Can you work these out from the model? Positions are in its coordinate system, mm. Face numbers are marked on the shaded views. Give positions to 0.01 mm unless a question says otherwise; leave off trailing zeros. Order: outer loops, then holes, each group sorted by start corner. A loop starts at its lowest first (then second) coordinate and runs counter-clockwise, first axis right, second up. Notation, with made-up numbers: (-5.5, -28.5) - (20.5, -28.5) arc R22 ccw to (20.5, -19.5) - close; hole circle Ø7 at (42, -25). An arc over 180 degrees is marked (long way). Use one line per item in the form item = value. Start each with the question number.
1) Suppose I cut it at A-A, the plane x = 0. Write out the boundary of the cut face in (y, z).
2) Suppose I cut it at B-B, the plane y = 43. Write out the boundary of the cut face in (x, z), and give its area (3 significant figures).
3) For pin 1 (2 mm diameter, centred on x = 5, y = 123, fed in from -Z); pin 2 (5 mm diameter, centred on y = 103.5, z = -5.5, fed in from -X), each with a flat end and sliding along its axis, tell me the tip position at first contact or that it passes through.
4) We'd pull the mould along Z, two halves only. Please class the marked faces 1 and 2: released by +Z, released by -Z, zero draft, split by the parting line, or undercut.
5) Suppose I cut it at C-C, the plane z = -2.5. Write out the boundary of the cut face in (x, y).
6) Please list where these lines run through material, in increasing order: probe 1 along X at (y, z) = (132, -0.25); probe 2 along Z at (x, y) = (-0.25, 47); probe 3 along X at (y, z) = (40, -1.5).
```python
from build123d import *

# Parameters (mm, degrees)
SEMICIRCULAR_TUBE_DEPTH = 170
FILLET_EDGES_R          = 1.1


with BuildPart() as part:
    # Sketch1 → semicircular tube (new body)
    with BuildSketch(Plane(origin=(0, 0, 0), x_dir=(1, 0, 0), z_dir=(0, 1, 0))):
        with BuildLine():
            Line((-9.35, 0), (-9.35, -3.5))
            Line((-9.35, -3.5), (9.35, -3.5))
            Line((9.35, -3.5), (9.35, 0))
            ThreePointArc((9.35, 0), (0, 9.35), (-9.35, 0))
        make_face()
        with BuildLine():
            Line((-6.35, 0), (6.35, 0))
            ThreePointArc((6.35, 0), (0, 6.35), (-6.35, 0))
        make_face(mode=Mode.SUBTRACT)
    extrude(amount=SEMICIRCULAR_TUBE_DEPTH)

    # fillet edges
    fillet_edges_edges = [part.edges().sort_by_distance(p)[0] for p in [
        (9.35, 85, 3.5),
        (-9.35, 85, 3.5),
    ]]
    fillet(fillet_edges_edges, radius=FILLET_EDGES_R)


solid = part.part
```
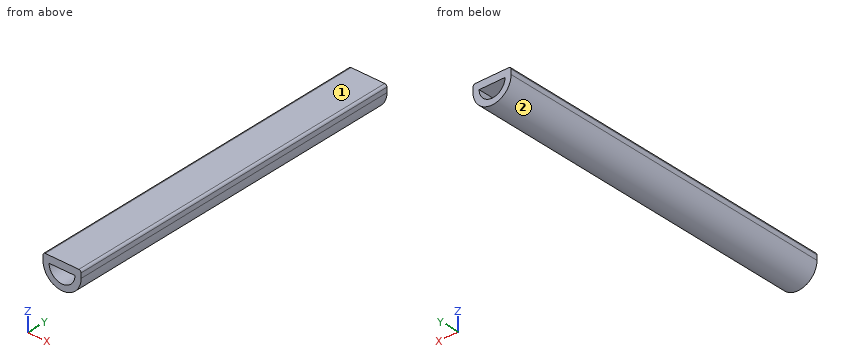
Result sheet:
q1.outline = (0, -9.35) - (170, -9.35) - (170, -6.35) - (0, -6.35) - close; (0, 0) - (170, 0) - (170, 3.5) - (0, 3.5) - close
q2.outline = (-9.35, 0) arc R9.35 ccw to (9.35, 0) - (9.35, 2.4) arc R1.1 ccw to (8.25, 3.5) - (-8.25, 3.5) arc R1.1 ccw to (-9.35, 2.4) - close; hole (-6.35, 0) arc R6.35 ccw to (6.35, 0) - close
q2.area = 139 mm²
q3.pin_1 = -8.45
q3.pin_2 = -8.86
q4.face_1 = released by +Z
q4.face_2 = released by -Z
q5.outline = (-9.01, 0) - (-5.84, 0) - (-5.84, 170) - (-9.01, 170) - close; (5.84, 0) - (9.01, 0) - (9.01, 170) - (5.84, 170) - close
q6.probe_1 = -9.35 to -6.35, 6.35 to 9.35
q6.probe_2 = -9.35 to -6.35, 0 to 3.5
q6.probe_3 = -9.23 to -6.17, 6.17 to 9.23
